For this review, take the finished solid that the model builds, in its own axes (mm). Round coordinates to 2 decimals unless told otherwise and drop trailing zeros. Order: outer loops, then holes, each group sorted by start corner. A loop starts at its lowest first (then second) coordinate and runs counter-clockwise, first axis right, second up. Notation, with made-up numbers: M 62,67.5 L 103,67.5 A8 cw 103,78.5 Z; hole C 53.5,35.5 d9. An arc over 180 degrees is marked long. Answer as a JSON object with one key per item and string values.
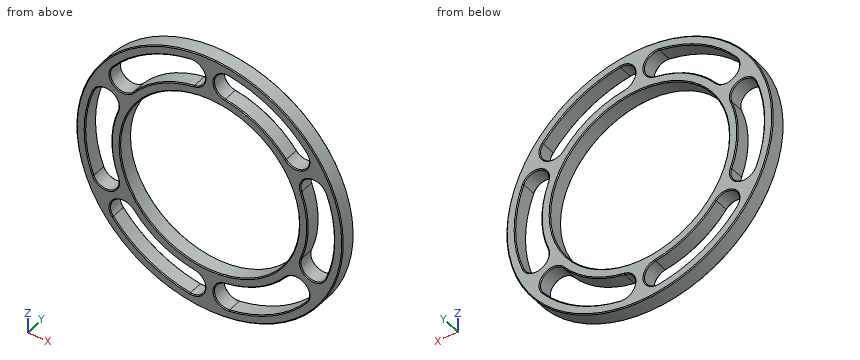
from build123d import *

# Parameters (mm, degrees)
SKETCH1_W                    = 24.97495
SKETCH1_H                    = 9
CUT_EXTRUDE1_DEPTH           = 10
CHAMFER3_SIZE                = 0.5
CHAMFER4_SIZE                = 0.5
CIRPATTERN1_COUNT            = 6
CHAMFER4_OF_CIRPATTERN1_SIZE = 0.5


with BuildPart() as part:
    # Sketch1 → Revolve1 (revolve)
    with BuildSketch(Plane.XY, mode=Mode.PRIVATE) as revolve1_sk:
        with Locations((63.612525, 4.5)):
            Rectangle(SKETCH1_W, SKETCH1_H)
    revolve(revolve1_sk.sketch.rotate(Axis((0, 0, 0), (0, 1, 0)), 90), axis=Axis((0, 0, 0), (0, 1, 0)))

    # Sketch2 → Cut-Extrude1 (cut)
    with BuildSketch(Plane(origin=(0, 9, 0), x_dir=(1, 0, 0), z_dir=(0, 1, 0))):
        with BuildLine():
            ThreePointArc((-66.392272497, 25.441622447), (-71.1, 0), (-66.392272497, -25.441622447))
            ThreePointArc((-66.392272497, -25.441622447), (-56.721330267, -29.754097391), (-52.408855323, -20.083155161))
            ThreePointArc((-52.408855323, -20.083155161), (-56.12505, 0), (-52.408855323, 20.083155161))
            ThreePointArc((-52.408855323, 20.083155161), (-56.721330267, 29.754097391), (-66.392272497, 25.441622447))
        make_face()
    cut_extrude1 = extrude(amount=-CUT_EXTRUDE1_DEPTH, mode=Mode.SUBTRACT)

    # Chamfer3
    chamfer3_edges = [part.edges().sort_by_distance(p)[0] for p in [
        (0, 0, 76.1),
        (0, 9, 76.1),
        (0, 9, 51.12505),
        (0, 0, 51.12505),
    ]]
    chamfer(chamfer3_edges, length=CHAMFER3_SIZE)

    # Chamfer4
    chamfer4_edges = [part.edges().sort_by_distance(p)[0] for p in [
        (-71.1, 0, 0),
        (-56.721330267, 0, -29.754097391),
        (-56.721330267, 0, 29.754097391),
        (-56.12505, 0, 0),
        (-56.12505, 9, 0),
        (-71.1, 9, 0),
        (-56.721330267, 9, 29.754097391),
        (-56.721330267, 9, -29.754097391),
    ]]
    chamfer(chamfer4_edges, length=CHAMFER4_SIZE)

    # CirPattern1: Cut-Extrude1 ×6 about axis
    cirpattern1_axis = Axis((0, 0, 0), (0, 1, 0))
    for i in range(1, CIRPATTERN1_COUNT):
        add(cut_extrude1.rotate(cirpattern1_axis, i * 360 / CIRPATTERN1_COUNT), mode=Mode.SUBTRACT)

    # Chamfer4 of CirPattern1
    chamfer4_of_cirpattern1_edges = [part.edges().sort_by_distance(p)[0] for p in [
        (-35.55, 0, 61.574406209),
        (-54.12846934, 0, 34.245064252),
        (-2.592860926, 0, 63.999161643),
        (-28.062525, 0, 48.605719089),
        (-28.062525, 9, 48.605719089),
        (-35.55, 9, 61.574406209),
        (-2.592860926, 9, 63.999161643),
        (-54.12846934, 9, 34.245064252),
        (35.55, 0, 61.574406209),
        (2.592860926, 0, 63.999161643),
        (54.12846934, 0, 34.245064252),
        (28.062525, 0, 48.605719089),
        (28.062525, 9, 48.605719089),
        (35.55, 9, 61.574406209),
        (54.12846934, 9, 34.245064252),
        (2.592860926, 9, 63.999161643),
        (71.1, 0, 0),
        (56.721330267, 0, 29.754097391),
        (56.721330267, 0, -29.754097391),
        (56.12505, 0, 0),
        (56.12505, 9, 0),
        (71.1, 9, 0),
        (56.721330267, 9, -29.754097391),
        (56.721330267, 9, 29.754097391),
        (35.55, 0, -61.574406209),
        (54.12846934, 0, -34.245064252),
        (2.592860926, 0, -63.999161643),
        (28.062525, 0, -48.605719089),
        (28.062525, 9, -48.605719089),
        (35.55, 9, -61.574406209),
        (2.592860926, 9, -63.999161643),
        (54.12846934, 9, -34.245064252),
        (-35.55, 0, -61.574406209),
        (-2.592860926, 0, -63.999161643),
        (-54.12846934, 0, -34.245064252),
        (-28.062525, 0, -48.605719089),
        (-28.062525, 9, -48.605719089),
        (-35.55, 9, -61.574406209),
        (-54.12846934, 9, -34.245064252),
        (-2.592860926, 9, -63.999161643),
    ]]
    chamfer(chamfer4_of_cirpattern1_edges, length=CHAMFER4_OF_CIRPATTERN1_SIZE)


solid = part.part
1) Add section B-B on x = 0. State the section outline as (y, z) points, and give its area (3 significant figures).
Geometry check:
{"outline": "M 0,-75.6 L 0.5,-76.1 L 8.5,-76.1 L 9,-75.6 L 9,-51.63 L 8.5,-51.13 L 0.5,-51.13 L 0,-51.63 Z; M 0,51.63 L 0.5,51.13 L 8.5,51.13 L 9,51.63 L 9,75.6 L 8.5,76.1 L 0.5,76.1 L 0,75.6 Z", "area": "449 mm²"}
2) Add section C-C on z = 0. State how many separate pieces and enclosed holes the cut face has, and give its area (3 significant figures).
Geometry check:
{"separate pieces": "4", "enclosed holes": "0", "area": "178 mm²"}
3) For L1, parallel to X at y = 4, z = 0; L2, parallel to X at y = 6.5, z = -18; L3, parallel to X at y = 6.75, z = -63.5, list the stretches that pass through material, from the lowest coordinate up.
Geometry check:
{"L1": "x = -76.1 to -71.1, -56.13 to -51.13, 51.13 to 56.13, 71.1 to 76.1", "L2": "x = -73.94 to -68.78, -53.16 to -47.85, 47.85 to 53.16, 68.78 to 73.94", "L3": "x = -41.94 to -31.98, -2.53 to 2.53, 31.98 to 41.94"}
4) Insertion check: P1, Ø1, axis at y = 7, z = -54.5, coming from the -X side; P2, Ø3, axis at x = -43.5, y = 6, coming from the +Z side; P3, Ø5, axis at x = -53.5, y = 2.5, coming from the +Z side. Each pin has a flat end and moves straight along its axis. Give the tip position at first contact, or say it passes through.
Geometry check:
{"P1": "stops at x = -53.62", "P2": "stops at z = 63.46", "P3": "stops at z = 56.48"}
